Verification items for the finished model (mm, model axes). Coordinates: 2 decimals unless noted, no trailing zeros. Write each loop counter-clockwise with the first axis right and the second up, starting at its lowest first coordinate (ties: lowest second). Pieces come first, ordered by that corner, then holes. Notation, with made-up numbers: (49, -33.75) -> (83, -33.75) arc R27 cw to (83, -14.75) -> close; hole circle Ø10 at (54, -9). An arc over 180 degrees is marked (long way). Use a Markdown table: item, result. Add a question column.
from build123d import *

# Parameters (mm, degrees)
SKETCH1_R                                     = 406.4
BOSS_EXTRUDE1_DEPTH                           = 6.35
CSK_FOR_1_4_FLAT_HEAD_MACHINE_SCREW1_AT_COUNT = 2
CSK_FOR_1_4_FLAT_HEAD_MACHINE_SCREW1_AT_PITCH = 235.470949714
CSK_FOR_1_4_FLAT_HEAD_MACHINE_SCREW1_2_COUNT  = 2
CSK_FOR_1_4_FLAT_HEAD_MACHINE_SCREW1_2_PITCH  = 447.892362247
CSK_FOR_1_4_FLAT_HEAD_MACHINE_SCREW1_3_COUNT  = 2
CSK_FOR_1_4_FLAT_HEAD_MACHINE_SCREW1_3_PITCH  = 616.470949714
CSK_FOR_1_4_FLAT_HEAD_MACHINE_SCREW1_4_COUNT  = 2
CSK_FOR_1_4_FLAT_HEAD_MACHINE_SCREW1_4_PITCH  = 724.705065417
CSK_FOR_1_4_FLAT_HEAD_MACHINE_SCREW1_5_COUNT  = 2
CSK_FOR_1_4_FLAT_HEAD_MACHINE_SCREW1_5_PITCH  = 762
CSK_FOR_1_4_FLAT_HEAD_MACHINE_SCREW1_6_COUNT  = 2
CSK_FOR_1_4_FLAT_HEAD_MACHINE_SCREW1_6_PITCH  = 724.705065417
CSK_FOR_1_4_FLAT_HEAD_MACHINE_SCREW1_7_COUNT  = 2
CSK_FOR_1_4_FLAT_HEAD_MACHINE_SCREW1_7_PITCH  = 616.470949714
CSK_FOR_1_4_FLAT_HEAD_MACHINE_SCREW1_8_COUNT  = 2
CSK_FOR_1_4_FLAT_HEAD_MACHINE_SCREW1_8_PITCH  = 447.892362247
CSK_FOR_1_4_FLAT_HEAD_MACHINE_SCREW1_9_COUNT  = 2
CSK_FOR_1_4_FLAT_HEAD_MACHINE_SCREW1_9_PITCH  = 235.470949714
F_10_0_1935_DIAMETER_HOLE1_D                  = 4.9149
F_1_8_0_125_DIAMETER_HOLE1_D                  = 3.175


with BuildPart() as part:
    # Sketch1 → Boss-Extrude1 (new body)
    with BuildSketch(Plane(origin=(0, 0, 0), x_dir=(1, 0, 0), z_dir=(0, 1, 0))):
        Circle(SKETCH1_R)
    extrude(amount=BOSS_EXTRUDE1_DEPTH)

    # Sketch6 → CSK for 1/4 Flat Head Machine Screw1 (revolve, cut)
    with BuildSketch(Plane(origin=(-117.735474857, 6.35, -362.352532708), x_dir=(0, 0, 1), z_dir=(1, 0, 0))):
        Polygon((0, 0), (0, 6.35), (3.3782, 6.35), (3.3782, 3.520932584), (6.4389, 0), align=None)
    csk_for_1_4_flat_head_machine_screw1 = revolve(axis=Axis((-117.735474857, 12.7, -362.352532708), (0, -1, 0)), mode=Mode.SUBTRACT)

    # CSK for 1/4 Flat Head Machine Screw1 at: CSK for 1/4 Flat Head Machine Screw1 ×2
    with Locations(*[(i * CSK_FOR_1_4_FLAT_HEAD_MACHINE_SCREW1_AT_PITCH, 0, 0) for i in range(1, CSK_FOR_1_4_FLAT_HEAD_MACHINE_SCREW1_AT_COUNT)]):
        add(csk_for_1_4_flat_head_machine_screw1, mode=Mode.SUBTRACT)

    # CSK for 1_4 Flat Head Machine Screw1 2: CSK for 1/4 Flat Head Machine Screw1 ×2
    with Locations(*[Vector(0.951056516, 0, 0.309016994) * (i * CSK_FOR_1_4_FLAT_HEAD_MACHINE_SCREW1_2_PITCH) for i in range(1, CSK_FOR_1_4_FLAT_HEAD_MACHINE_SCREW1_2_COUNT)]):
        add(csk_for_1_4_flat_head_machine_screw1, mode=Mode.SUBTRACT)

    # CSK for 1_4 Flat Head Machine Screw1 3: CSK for 1/4 Flat Head Machine Screw1 ×2
    with Locations(*[Vector(0.809016994, 0, 0.587785252) * (i * CSK_FOR_1_4_FLAT_HEAD_MACHINE_SCREW1_3_PITCH) for i in range(1, CSK_FOR_1_4_FLAT_HEAD_MACHINE_SCREW1_3_COUNT)]):
        add(csk_for_1_4_flat_head_machine_screw1, mode=Mode.SUBTRACT)

    # CSK for 1_4 Flat Head Machine Screw1 4: CSK for 1/4 Flat Head Machine Screw1 ×2
    with Locations(*[Vector(0.587785252, 0, 0.809016994) * (i * CSK_FOR_1_4_FLAT_HEAD_MACHINE_SCREW1_4_PITCH) for i in range(1, CSK_FOR_1_4_FLAT_HEAD_MACHINE_SCREW1_4_COUNT)]):
        add(csk_for_1_4_flat_head_machine_screw1, mode=Mode.SUBTRACT)

    # CSK for 1_4 Flat Head Machine Screw1 5: CSK for 1/4 Flat Head Machine Screw1 ×2
    with Locations(*[Vector(0.309016994, 0, 0.951056516) * (i * CSK_FOR_1_4_FLAT_HEAD_MACHINE_SCREW1_5_PITCH) for i in range(1, CSK_FOR_1_4_FLAT_HEAD_MACHINE_SCREW1_5_COUNT)]):
        add(csk_for_1_4_flat_head_machine_screw1, mode=Mode.SUBTRACT)

    # CSK for 1_4 Flat Head Machine Screw1 6: CSK for 1/4 Flat Head Machine Screw1 ×2
    with Locations(*[(0, 0, i * CSK_FOR_1_4_FLAT_HEAD_MACHINE_SCREW1_6_PITCH) for i in range(1, CSK_FOR_1_4_FLAT_HEAD_MACHINE_SCREW1_6_COUNT)]):
        add(csk_for_1_4_flat_head_machine_screw1, mode=Mode.SUBTRACT)

    # CSK for 1_4 Flat Head Machine Screw1 7: CSK for 1/4 Flat Head Machine Screw1 ×2
    with Locations(*[Vector(-0.309016994, 0, 0.951056516) * (i * CSK_FOR_1_4_FLAT_HEAD_MACHINE_SCREW1_7_PITCH) for i in range(1, CSK_FOR_1_4_FLAT_HEAD_MACHINE_SCREW1_7_COUNT)]):
        add(csk_for_1_4_flat_head_machine_screw1, mode=Mode.SUBTRACT)

    # CSK for 1_4 Flat Head Machine Screw1 8: CSK for 1/4 Flat Head Machine Screw1 ×2
    with Locations(*[Vector(-0.587785252, 0, 0.809016994) * (i * CSK_FOR_1_4_FLAT_HEAD_MACHINE_SCREW1_8_PITCH) for i in range(1, CSK_FOR_1_4_FLAT_HEAD_MACHINE_SCREW1_8_COUNT)]):
        add(csk_for_1_4_flat_head_machine_screw1, mode=Mode.SUBTRACT)

    # CSK for 1_4 Flat Head Machine Screw1 9: CSK for 1/4 Flat Head Machine Screw1 ×2
    with Locations(*[Vector(-0.809016994, 0, 0.587785252) * (i * CSK_FOR_1_4_FLAT_HEAD_MACHINE_SCREW1_9_PITCH) for i in range(1, CSK_FOR_1_4_FLAT_HEAD_MACHINE_SCREW1_9_COUNT)]):
        add(csk_for_1_4_flat_head_machine_screw1, mode=Mode.SUBTRACT)

    # #10 (0.1935) Diameter Hole1 (through all)
    with Locations(Plane(origin=(0, 6.35, 0), x_dir=(1, 0, 0), z_dir=(0, 1, 0))):
        with Locations((0, -120.2563), (120.2563, 0), (0, 120.2563), (-120.2563, 0)):
            Hole(F_10_0_1935_DIAMETER_HOLE1_D / 2)

    # 1/8 (0.125) Diameter Hole1 (through all)
    with Locations(Plane(origin=(0, 6.35, 0), x_dir=(1, 0, 0), z_dir=(0, 1, 0))):
        with Locations((-406.4, 0), (406.4, 0)):
            Hole(F_1_8_0_125_DIAMETER_HOLE1_D / 2)


solid = part.part
1) Cross-section at A-A on y = 4.75. Give the number of separate pieces and of enclosed holes in the cut face, then the cut area to 3 significant figures.
2) Cross-section at B-B on x = 266.5. Record the boundary of the cut face in (y, z).
3) Thickness scan on L1, parallel to Z at x = 0, y = 1.5; L2, parallel to Z at x = 119, y = 1.75; L3, parallel to Z at x = 37, y = 3.5. Record the ranges inside material, lowest first.
4) Release check for a two-part mould opening along Z. For faces 1 (the face through (-8.914, 3.131, 406.302)), 2 (the face through (8.914, 3.131, -406.302)), 3 (the face through (-6, 6.35, -6)) record: released by +Z, released by -Z, zero draft, split by the parting line, or undercut.
5) Cross-section at C-C on x = 98.5. Record the boundary of the cut face in (y, z).
6) Gauge pin test, flat ends, axial feed: pin 1 (3 mm diameter, centred on y = 5.5, z = -257.5, fed in from +X); pin 2 (1.5 mm diameter, centred on x = 98.5, y = 5.5, fed in from -Z); pin 3 (9 mm diameter, centred on x = -308.24, z = 223.95, fed in from +Y). Record the tip position at first contact, or that the pin passes through.
Returned:
| question | item | result |
|---|---|---|
| 1 | separate pieces | 1 |
| 1 | enclosed holes | 14 |
| 1 | area | 518,000 mm² |
| 2 | outline | (0, -306.82) -> (6.35, -306.82) -> (6.35, 306.82) -> (0, 306.82) -> close |
| 3 | L1 | z = -406.4 to -122.71, -117.8 to 117.8, 122.71 to 406.4 |
| 3 | L2 | z = -388.59 to -365.49, -359.22 to -2.11, 2.11 to 359.22, 365.49 to 388.59 |
| 3 | L3 | z = -404.71 to 404.71 |
| 4 | face 1 | released by +Z |
| 4 | face 2 | released by -Z |
| 4 | face 3 | zero draft |
| 5 | outline | (0, -394.28) -> (6.35, -394.28) -> (6.35, 394.28) -> (0, 394.28) -> close |
| 6 | pin 1 | stops at x = 315.63 |
| 6 | pin 2 | stops at z = -394.47 |
| 6 | pin 3 | stops at y = 4.13 |
